Check sheet for the modelled part. Datum: model origin and axes. Units: mm. Give positions to 0.01 mm unless a question says otherwise; leave off trailing zeros. Loops run counter-clockwise (first coordinate to the right, second up) from the corner with the lowest first, then second, coordinate; pieces in that order, holes last.
```python
from build123d import *

# Parameters (mm, degrees)
ESQUISSE1_R             = 1.558671709
ESQUISSE1_R_2           = 1.510734584
BOSS_EXTRU_1_DEPTH      = 11
ESQUISSE2_W             = 30
ESQUISSE2_H             = 7.376780582
ENL_V_MAT_EXTRU_1_DEPTH = 10


with BuildPart() as part:
    # Esquisse1 → Boss.-Extru.1 (new body)
    with BuildSketch(Plane.XY):
        with BuildLine():
            Line((-27.586844937, 4.788639913), (15.827697586, 16.628297741))
            ThreePointArc((15.827697586, 16.628297741), (20.43658301, 13.99456085), (17.802846119, 9.385675426))
            Line((17.802846119, 9.385675426), (-25.611696404, -2.453982402))
            ThreePointArc((-25.611696404, -2.453982402), (-30.220581828, 0.179754489), (-27.586844937, 4.788639913))
        make_face()
        with Locations((-26.599270671, 1.167328755)):
            Circle(ESQUISSE1_R, mode=Mode.SUBTRACT)
        with Locations((16.815271853, 13.006986583)):
            Circle(ESQUISSE1_R_2, mode=Mode.SUBTRACT)
    extrude(amount=BOSS_EXTRU_1_DEPTH)

    # Esquisse2 → Enlèv. mat.-Extru.1 (cut)
    with BuildSketch(Plane(origin=(-3.125175124, 11.4596258, 0), x_dir=(0.9647676116315722, 0.2631035072869839, 0), z_dir=(-0.2631035072869839, 0.9647676116315722, 0))):
        with Locations((-18.354986546, -7.311609709)):
            Rectangle(ESQUISSE2_W, ESQUISSE2_H)
    extrude(amount=-ENL_V_MAT_EXTRU_1_DEPTH, mode=Mode.SUBTRACT)


solid = part.part
```
(1) Material ranges on line 1 (Z direction, x = -25.5, y = 0); line 2 (Y direction, x = 1, z = 2.75); line 3 (Y direction, x = -0.5, z = 7.5), recorded low to high.
(2) Release check for a two-part mould opening along Y. For faces 1 (the face through (-5.39, 7.01, 7.36)), 2 (the face through (-30.198, 0.1, 1.786)), 3 (the face through (15.616, 12.088, 5.423)), 4 (the face through (-25.1, 1.6, 1.8)) record: pulls with the +Y half, pulls with the -Y half, needs draft (parallel to the pull), parting line crosses it, or undercut.
(3) Gauge pin test, flat ends, axial feed: pin 1 Ø2 at (x, z) = (-6, 6.5) entering from +Y; pin 2 Ø3.5 at (x, y) = (16.82, 13.01) entering from +Z; pin 3 Ø6 at (x, y) = (-9, 1) entering from +Z; pin 4 Ø3 at (x, z) = (5, 8.5) entering from +Y. Record the tip position at first contact, or that the pin passes through.
(4) Section check A-A on y = 12. Record the boundary of the cut face in (x, z).
(5) Section check D-D on z = 1.25. Record the boundary of the cut face in (x, y), plus the area to 3 significant figures.
(6) Section check C-C on x = -27. Record the boundary of the cut face in (y, z).
(7) Section check B-B on z = 9.25. Record the boundary of the cut face in (x, y).
Computed values:
1. line 1: z = 0 to 3.62
1. line 2: y = 4.8 to 12.58
1. line 3: y = 4.39 to 12.18
2. face 1: pulls with the -Y half
2. face 2: parting line crosses it
2. face 3: undercut
2. face 4: undercut
3. pin 1: stops at y = 10.95
3. pin 2: stops at z = 11
3. pin 3: stops at z = 3.62
3. pin 4: stops at y = 14.08
4. outline: (-1.14, 0) - (15.69, 0) - (15.69, 11) - (-1.14, 11) - close; (17.94, 0) - (20.43, 0) - (20.43, 11) - (17.94, 11) - close
5. outline: (-27.59, 4.79) arc R3.75 ccw to (-25.61, -2.45) - (17.8, 9.39) arc R3.75 ccw to (15.83, 16.63) - close; hole circle Ø3.12 at (-26.6, 1.17); hole circle Ø3.02 at (16.82, 13.01)
5. area: 367 mm2
6. outline: (-2.56, 0) - (-0.34, 0) - (-0.34, 3.62) - (-2.56, 3.62) - close; (2.67, 0) - (4.95, 0) - (4.95, 3.62) - (2.67, 3.62) - close
7. outline: (-6.36, 10.58) - (-4.39, 3.33) - (17.8, 9.39) arc R3.75 ccw to (15.83, 16.63) - close; hole circle Ø3.02 at (16.82, 13.01)
